Read the model definition and answer for the solid it produces. Units are mm, in the model's axes. Coordinates: 2 decimals unless noted, no trailing zeros.
from build123d import *

# Parameters (mm, degrees)
BOSS_EXTRUDE1_DEPTH = 2.54
CUT_EXTRUDE1_DEPTH  = 126.848428748
LPATTERN1_DEPTH     = 2.54


# Read off the part's stored shape, not the designer's step: LPattern1
with BuildPart() as part:
    # Sketch1 → Boss-Extrude1 (new body)
    with BuildSketch(Plane.XY):
        with BuildLine():
            Line((0, 0), (80.01, 0))
            add(Edge.make_bspline(
                [(80.01, 0), (96.839490245, 38.288168981), (98.456742521, 78.343125)],
                knots=[0, 0, 0, 0.824657213, 0.824657213, 0.824657213], degree=2))
            Line((98.456742521, 78.343125), (18.446742521, 78.343125))
            add(Edge.make_bspline(
                [(0, 0), (16.829490245, 38.288168981), (18.446742521, 78.343125)],
                knots=[0, 0, 0, 0.824657213, 0.824657213, 0.824657213], degree=2))
        make_face()
    extrude(amount=BOSS_EXTRUDE1_DEPTH)

    # Sketch2 → Cut-Extrude1 (cut, through all)
    with BuildSketch(Plane.XY.offset(2.54)):
        with BuildLine():
            Line((10.043267201, 7.62), (74.813267201, 7.62))
            ThreePointArc((74.813267201, 7.62), (76.718267201, 5.715), (74.813267201, 3.81))
            Line((74.813267201, 3.81), (10.043267201, 3.81))
            ThreePointArc((10.043267201, 3.81), (8.138267201, 5.715), (10.043267201, 7.62))
        make_face()
    extrude(amount=-CUT_EXTRUDE1_DEPTH, mode=Mode.SUBTRACT)

    # LPattern1 outline → LPattern1 (cut)
    with BuildSketch(Plane.XY):
        with BuildLine():
            Line((77.770374016, 15.24), (13.000374016, 15.24))
            ThreePointArc((13.000374016, 15.24), (11.095374016, 13.335), (13.000374016, 11.43))
            Line((13.000374016, 11.43), (77.770374016, 11.43))
            ThreePointArc((77.770374016, 11.43), (79.675374016, 13.335), (77.770374016, 15.24))
        make_face()
        with BuildLine():
            Line((80.418314493, 22.86), (15.648314493, 22.86))
            ThreePointArc((15.648314493, 22.86), (13.743314493, 20.955), (15.648314493, 19.05))
            Line((15.648314493, 19.05), (80.418314493, 19.05))
            ThreePointArc((80.418314493, 19.05), (82.323314493, 20.955), (80.418314493, 22.86))
        make_face()
        with BuildLine():
            Line((82.761233407, 30.48), (17.991233408, 30.48))
            ThreePointArc((17.991233408, 30.48), (16.086233408, 28.575), (17.991233408, 26.67))
            Line((17.991233408, 26.67), (82.761233407, 26.67))
            ThreePointArc((82.761233407, 26.67), (84.666233407, 28.575), (82.761233407, 30.48))
        make_face()
        with BuildLine():
            Line((84.803183747, 38.1), (20.033183747, 38.1))
            ThreePointArc((20.033183747, 38.1), (18.128183747, 36.195), (20.033183747, 34.29))
            Line((20.033183747, 34.29), (84.803183747, 34.29))
            ThreePointArc((84.803183747, 34.29), (86.708183747, 36.195), (84.803183747, 38.1))
        make_face()
        with BuildLine():
            Line((86.548129526, 45.72), (21.778129526, 45.72))
            ThreePointArc((21.778129526, 45.72), (19.873129526, 43.815), (21.778129526, 41.91))
            Line((21.778129526, 41.91), (86.548129526, 41.91))
            ThreePointArc((86.548129526, 41.91), (88.453129526, 43.815), (86.548129526, 45.72))
        make_face()
        with BuildLine():
            Line((87.999948503, 53.34), (23.229948503, 53.34))
            ThreePointArc((23.229948503, 53.34), (21.324948503, 51.435), (23.229948503, 49.53))
            Line((23.229948503, 49.53), (87.999948503, 49.53))
            ThreePointArc((87.999948503, 49.53), (89.904948503, 51.435), (87.999948503, 53.34))
        make_face()
        with BuildLine():
            Line((89.16243478, 60.96), (24.39243478, 60.96))
            ThreePointArc((24.39243478, 60.96), (22.48743478, 59.055), (24.39243478, 57.15))
            Line((24.39243478, 57.15), (89.16243478, 57.15))
            ThreePointArc((89.16243478, 57.15), (91.06743478, 59.055), (89.16243478, 60.96))
        make_face()
        with BuildLine():
            Line((90.039301311, 68.58), (25.269301311, 68.58))
            ThreePointArc((25.269301311, 68.58), (23.364301311, 66.675), (25.269301311, 64.77))
            Line((25.269301311, 64.77), (90.039301311, 64.77))
            ThreePointArc((90.039301311, 64.77), (91.944301311, 66.675), (90.039301311, 68.58))
        make_face()
        with BuildLine():
            Line((90.634182309, 76.2), (25.864182309, 76.2))
            ThreePointArc((25.864182309, 76.2), (23.959182309, 74.295), (25.864182309, 72.39))
            Line((25.864182309, 72.39), (90.634182309, 72.39))
            ThreePointArc((90.634182309, 72.39), (92.539182309, 74.295), (90.634182309, 76.2))
        make_face()
    extrude(amount=LPATTERN1_DEPTH, mode=Mode.SUBTRACT)


solid = part.part
Q1. Determine the mould class of faces 1 (the face through (39, 0, 1)), 2 (the face through (21.325, 51.477, 1.252)) for opening direction X: +X half, -X half, draft (parallel to the pull), parting line (faces both ways), or undercut.
Findings below:
face 1: draft
face 2: undercut
Q2. A flat-ended cylindrical pin translates along its axis: pin 1 Ø0.8 at (x, z) = (45, 1.5) entering from -Y. Find the tip coordinate at first contact, or state that the pin passes through.
Findings below:
pin 1: stops at y = 0
Q3. Straight lines are drawn through the part: probe 1 along Y at (x, z) = (19, 0.55); probe 2 along X at (y, z) = (13, 2.15); probe 3 along X at (y, z) = (68, 1.1). For each, find the intervals that lie inside material, in ascending order.
Findings below:
probe 1: y = 0 to 3.81, 7.62 to 11.43, 15.24 to 19.05, 22.86 to 26.67, 30.48 to 34.59, 37.8 to 78.34
probe 2: x = 5.26 to 11.13, 79.65 to 85.27
probe 3: x = 17.77 to 23.9, 91.41 to 97.78
Q4. A cutting plane is placed at A-A (z = 1.4). Count the separate pieces of the cut face and the enclosed holes in it, then the cut area to 3 significant figures.
Findings below:
separate pieces: 1
enclosed holes: 10
area: 3,690 mm2
